The figure shows three views and two pictorial views of one solid part (mm, origin at its lowest corner). Answer the questions. A direction names the side the tool comes from. Give positions to 0.01 mm unless a question says otherwise; leave off trailing zeros. Write each loop counter-clockwise with the first axis right and the second up, starting at its lowest first coordinate (ties: lowest second). Pieces come first, ordered by that corner, then holes. Notation, with made-up numbers: M -18.75,89 L 26.25,89 A34 cw 26.25,120 Z; hole C 44.25,21.5 d10. An arc over 180 degrees is marked long. Answer as CSV lines item,"result". Start each with the question number.
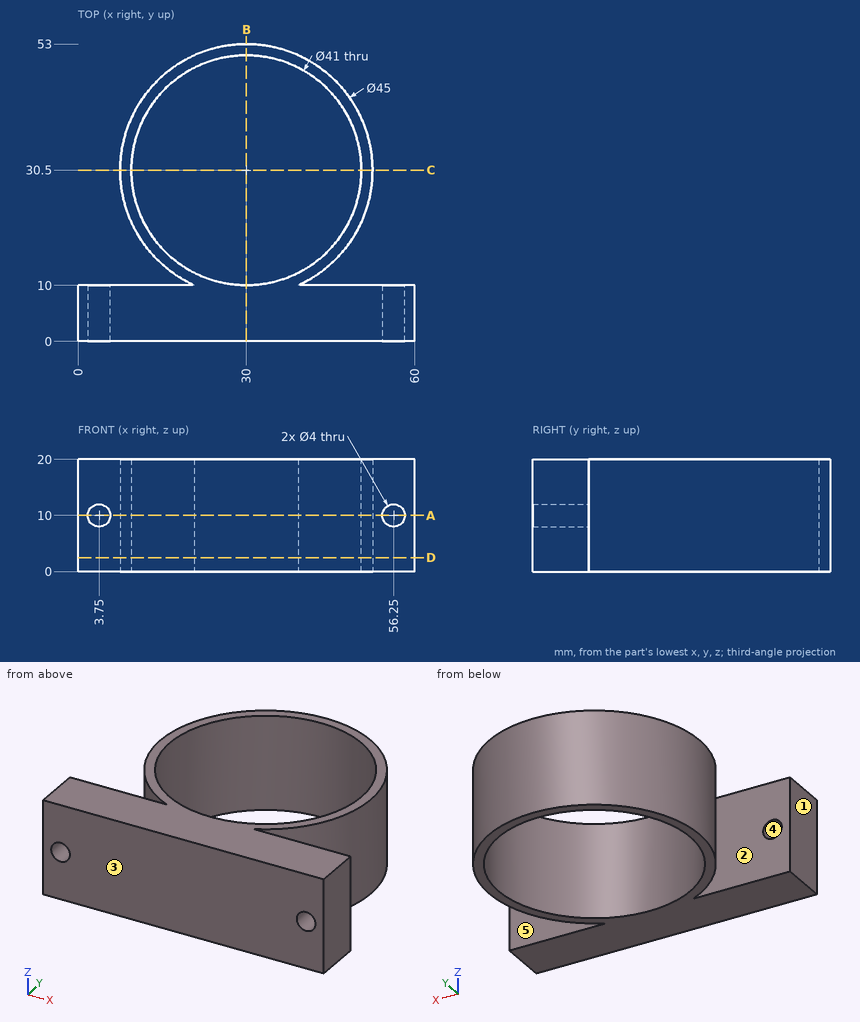
1. Determine the mould class of the marked faces 3, 4 and 5 for opening direction Y: +Y half, -Y half, draft (parallel to the pull), parting line (faces both ways), or undercut.
2. Find section D-D on z = 2.5. Determine the outline of the cut face in (x, y), then the cut area to 3 significant figures.
3. Find section A-A on z = 10. Determine the outline of the cut face in (x, y), then the cut area to 3 significant figures.
4. Given pin 1 (2.5 mm diameter, centred on x = 56.25, z = 10, fed in from +Y); pin 2 (8 mm diameter, centred on y = 19.5, z = 7.5, fed in from -X); pin 3 (2 mm diameter, centred on y = 11.5, z = 11.5, fed in from +X); pin 4 (12 mm diameter, centred on y = 32, z = 8, fed in from -X), each flat-ended and moving along its own axis, determine where each tip first touches the part or whether it passes through.
5. For the marked faces 1 and 2, determine the directions among +Z, -Z, +X, -X, +Y, -Y from which every point of the face is accessible in a straight line to the end or side of a thin tool.
6. Find section B-B on x = 30. Determine the outline of the cut face in (y, z), then the cut area to 3 significant figures.
7. Find the intervals of material crossed by line 1 (Z direction, x = 56.25, y = 3); line 2 (Y direction, x = 45.5, z = 14.5); line 3 (X direction, y = 30.5, z = 8.25), in increasing order. Write a range as [from, to].
8. Find section C-C on y = 30.5. Determine the outline of the cut face in (x, z).
Computed:
1,face 3,"-Y half"
1,face 4,"draft"
1,face 5,"undercut"
2,outline,"M 0,0 L 60,0 L 60,10 L 39.27,10 A22.5 ccw long 20.73,10 L 0,10 Z; hole C 30,30.5 d41"
2,area,"845 mm^2"
3,outline,"M 0,0 L 1.75,0 L 1.75,10 L 0,10 Z; M 5.75,0 L 54.25,0 L 54.25,10 L 39.27,10 A22.5 ccw long 20.73,10 L 5.75,10 Z; M 58.25,0 L 60,0 L 60,10 L 58.25,10 Z; hole C 30,30.5 d41"
3,area,"765 mm^2"
4,pin 1,"passes through"
4,pin 2,"stops at x = 8.62"
4,pin 3,"stops at x = 43.5"
4,pin 4,"stops at x = 7.5"
5,face 1,"+Z, -Z, -X, +Y, -Y"
5,face 2,"+Z, -Z, -X"
6,outline,"M 0,0 L 10,0 L 10,20 L 0,20 Z; M 51,0 L 53,0 L 53,20 L 51,20 Z"
6,area,"240 mm^2"
7,line 1,"z = [0, 8], [12, 20]"
7,line 2,"y = [0, 10], [14.19, 17.08], [43.92, 46.81]"
7,line 3,"x = [7.5, 9.5], [50.5, 52.5]"
8,outline,"M 7.5,0 L 9.5,0 L 9.5,20 L 7.5,20 Z; M 50.5,0 L 52.5,0 L 52.5,20 L 50.5,20 Z"
